Input: part model. Units: mm. Frame: model coordinates. A direction names the side the tool comes from. Round coordinates to 2 decimals unless told otherwise and drop trailing zeros. Loops run counter-clockwise (first coordinate to the right, second up) from the corner with the lowest first, then second, coordinate; pieces in that order, holes last. Notation, with made-up numbers: (12.25, -16.5) - (40.25, -16.5) arc R31 cw to (40.25, 22.5) - close; hole circle Ø8 at (-7, 40). An arc over 180 degrees is marked (long way). Use CSV: the item, a comma, the result in double quotes. Start each with the question number.
1. Pin query (flat end, axial travel): P1, Ø3, axis at y = 2, z = -70.5, coming from the +X side; P2, Ø1.5, axis at x = 1.5, y = 2, coming from the -Z side; P3, Ø1.9, axis at x = 26.32, z = -119.36, coming from the +Y side; P4, Ø3.5, axis at x = 19.34, z = -219.34, coming from the -Y side. Return the tip coordinate at first contact, or that it passes through.
2. Cut plane B-B (y = 1.5). Give the number of separate pieces and of enclosed holes in the cut face, and give its area (3 significant figures).
3. Material intervals for probe 1 along X at (y, z) = (3, -78); probe 2 along Z at (x, y) = (-11, 4.25); probe 3 along Z at (x, y) = (16.5, 2), sorted ascending. Write a range as from..to.
4. Cut plane C-C (z = -136.5). Return loops of the section in (x, y), and give its area (3 significant figures).
5. Access query for faces 1 (the flat face through (17.5, 3, -76)), 2 (the flat face through (0, 6.35, -106)). Directions: +Z, -Z, +X, -X, +Y, -Y. A direction counts if a zero-diameter tool reaches every point of the face in a straight line with its end or side. Return the directions, or none.
6. Cut plane D-D (z = -16). Return loops of the section in (x, y).
7. Pull-direction query (X, two-part tool) for faces 3 (the flat face through (-31.29, 3.13, -100.73)), 4 (the cylindrical face through (-0.605, 3.131, 27.493)), 5 (the flat face through (0, 3, -154)); classes: +X half, -X half, draft (parallel to the pull), parting line (faces both ways), or undercut.
8. Cut plane A-A (x = 0). Return loops of the section in (y, z), and give its area (3 significant figures).
```python
from build123d import *

# Parameters (mm, degrees)
BOSS_EXTRUDE1_DEPTH     = 6.35
SKETCH2_R               = 2.6
CUT_EXTRUDE1_DEPTH      = 238.676928834
ESQUISSE3_R             = 21
ENL_V_MAT_EXTRU_2_DEPTH = 238.676928834
ESQUISSE7_R             = 1.5
ENL_V_MAT_EXTRU_3_DEPTH = 238.676928834
CUT_EXTRUDE2_DEPTH      = 238.676928834
SKETCH5_R               = 1.625
CUT_EXTRUDE3_DEPTH      = 238.676928834
CUT_EXTRUDE5_DEPTH      = 238.676928834


with BuildPart() as part:
    # Sketch1 → Boss-Extrude1 (new body)
    with BuildSketch(Plane(origin=(0, 0, 0), x_dir=(1, 0, 0), z_dir=(0, 1, 0))):
        with BuildLine():
            Line((27.5, 0), (34.975254116, 198.684097441))
            ThreePointArc((34.975254116, 198.684097441), (0, 235), (-34.975254116, 198.684097441))
            Line((-34.975254116, 198.684097441), (-27.5, 0))
            ThreePointArc((-27.5, 0), (0, -27.5), (27.5, 0))
        make_face()
    extrude(amount=BOSS_EXTRUDE1_DEPTH)

    # Sketch2 → Cut-Extrude1 (cut, through all)
    with BuildSketch(Plane(origin=(0, 6.35, 0), x_dir=(1, 0, 0), z_dir=(0, 1, 0))):
        with Locations(Location((0, 0, 0), (0, 0, 270))):
            Circle(SKETCH2_R)
    extrude(amount=-CUT_EXTRUDE1_DEPTH, mode=Mode.SUBTRACT)

    # Esquisse3 → Enlèv. mat.-Extru.2 (cut, through all)
    with BuildSketch(Plane(origin=(0, 6.35, 0), x_dir=(1, 0, 0), z_dir=(0, 1, 0))):
        with Locations(Location((0, 200, 0), (0, 0, 270))):
            Circle(ESQUISSE3_R)
    extrude(amount=-ENL_V_MAT_EXTRU_2_DEPTH, mode=Mode.SUBTRACT)

    # Esquisse7 → Enlèv. mat.-Extru.3 (cut, through all)
    with BuildSketch(Plane(origin=(0, 6.35, 0), x_dir=(1, 0, 0), z_dir=(0, 1, 0))):
        with Locations(Location((-19.339370465, 219.339370465, 0), (0, 0, 270))):
            Circle(ESQUISSE7_R)
        with Locations(Location((19.339370465, 219.339370465, 0), (0, 0, 270))):
            Circle(ESQUISSE7_R)
        with Locations(Location((19.339370465, 180.660629535, 0), (0, 0, 270))):
            Circle(ESQUISSE7_R)
        with Locations(Location((-19.339370465, 180.660629535, 0), (0, 0, 270))):
            Circle(ESQUISSE7_R)
    extrude(amount=-ENL_V_MAT_EXTRU_3_DEPTH, mode=Mode.SUBTRACT)

    # Sketch3 → Cut-Extrude2 (cut, through all)
    with BuildSketch(Plane(origin=(0, 6.35, 0), x_dir=(1, 0, 0), z_dir=(0, 1, 0))):
        Polygon((21.15, 149.828069991), (21.15, 115.871930009), (16.978069991, 111.7), (-16.978069991, 111.7), (-21.15, 115.871930009), (-21.15, 149.828069991), (-16.978069991, 154), (16.978069991, 154), align=None)
    extrude(amount=-CUT_EXTRUDE2_DEPTH, mode=Mode.SUBTRACT)

    # Sketch5 → Cut-Extrude3 (cut, through all)
    with BuildSketch(Plane(origin=(0, 6.35, 0), x_dir=(1, 0, 0), z_dir=(0, 1, 0))):
        with Locations(Location((-27.331724457, 146.340455159, 0), (0, 0, 270))):
            Circle(SKETCH5_R)
        with Locations(Location((-26.316599626, 119.359544841, 0), (0, 0, 270))):
            Circle(SKETCH5_R)
    cut_extrude3 = extrude(amount=-CUT_EXTRUDE3_DEPTH, mode=Mode.SUBTRACT)

    # Mirror1: Cut-Extrude3 across plane
    add(cut_extrude3.mirror(Plane(origin=(0, 0, 0), x_dir=(0, 0, 1), z_dir=(1, 0, 0))), mode=Mode.SUBTRACT)

    # Sketch8 → Cut-Extrude5 (cut, through all)
    with BuildSketch(Plane(origin=(0, 6.35, 0), x_dir=(1, 0, 0), z_dir=(0, 1, 0))):
        with BuildLine():
            Line((-12.5, 96.7), (-12.5, 56.7))
            ThreePointArc((-12.5, 56.7), (-15, 54.2), (-17.5, 56.7))
            Line((-17.5, 56.7), (-17.5, 96.7))
            ThreePointArc((-17.5, 96.7), (-15, 99.2), (-12.5, 96.7))
        make_face()
    cut_extrude5 = extrude(amount=-CUT_EXTRUDE5_DEPTH, mode=Mode.SUBTRACT)

    # Mirror2: Cut-Extrude5 across plane
    add(cut_extrude5.mirror(Plane(origin=(0, 0, 0), x_dir=(0, 0, 1), z_dir=(1, 0, 0))), mode=Mode.SUBTRACT)


solid = part.part
```
Established:
1,P1,"stops at x = 30.21"
1,P2,"stops at z = -234.99"
1,P3,"passes through"
1,P4,"stops at y = 0"
2,separate pieces,"1"
2,enclosed holes,"13"
2,area,"12,000 mm2"
3,probe 1,"x = -30.43..-17.5, -12.5..12.5, 17.5..30.43"
3,probe 2,"z = -233.23..-217.89, -182.11..-154, -111.7..25.2"
3,probe 3,"z = -230.87..-212.99, -187.01..-154, -111.7..-98.7, -54.7..22"
4,outline,"(-32.64, 0) - (-21.15, 0) - (-21.15, 6.35) - (-32.64, 6.35) - close; (21.15, 0) - (32.64, 0) - (32.64, 6.35) - (21.15, 6.35) - close"
4,area,"146 mm2"
5,face 1,"+Y, -Y"
5,face 2,"+Z, -Z, +X, -X, +Y"
6,outline,"(-28.1, 0) - (28.1, 0) - (28.1, 6.35) - (-28.1, 6.35) - close"
7,face 3,"-X half"
7,face 4,"parting line"
7,face 5,"undercut"
8,outline,"(0, -235) - (6.35, -235) - (6.35, -221) - (0, -221) - close; (0, -179) - (6.35, -179) - (6.35, -154) - (0, -154) - close; (0, -111.7) - (6.35, -111.7) - (6.35, -2.6) - (0, -2.6) - close; (0, 2.6) - (6.35, 2.6) - (6.35, 27.5) - (0, 27.5) - close"
8,area,"1,100 mm2"
